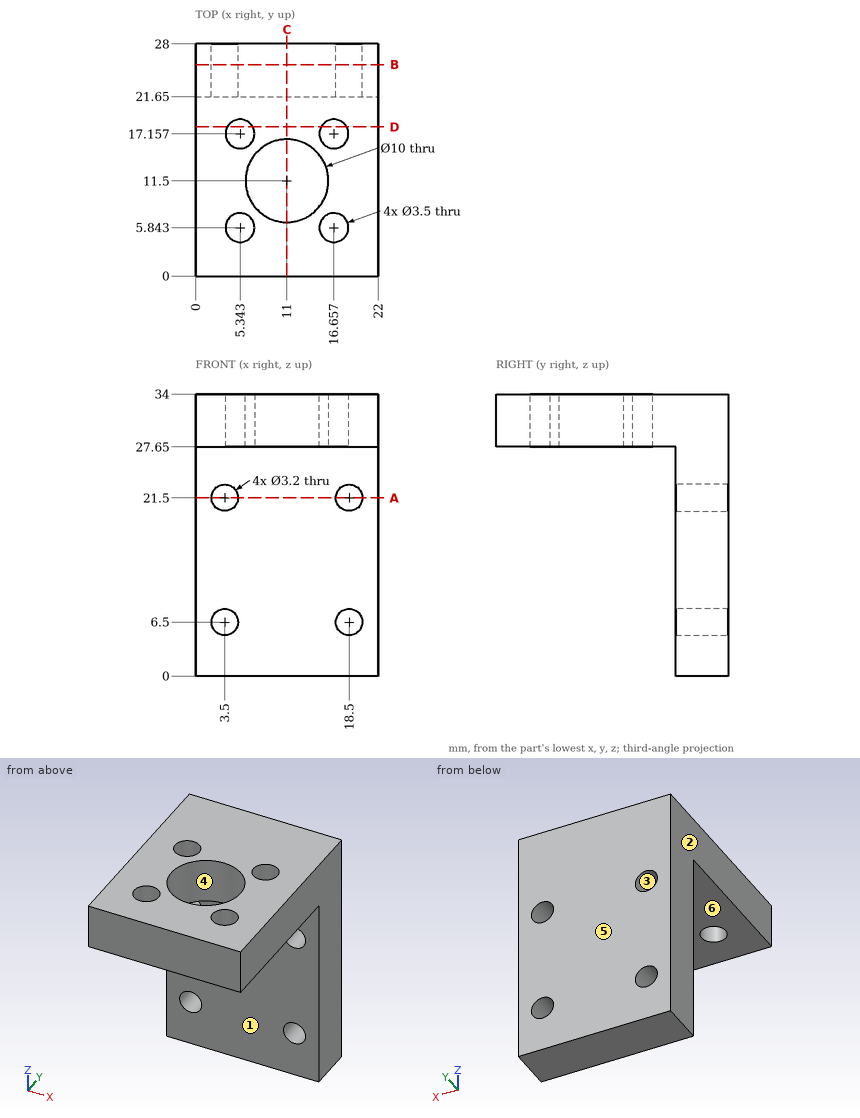
Answer from the drawing. Dimensions are ordinates in mm from the lowest x, y and z of the part. A direction names the side the tool comes from. Coordinates: 2 decimals unless noted, no trailing zeros. Loops run counter-clockwise (first coordinate to the right, second up) from the corner with the lowest first, then second, coordinate; pieces in that order, holes last. Notation, with made-up numbers: (57, 69) - (93, 69) arc R32 ccw to (93, 108) - close; hole circle Ø9 at (41.25, 15). An arc over 180 degrees is marked (long way). Use a Markdown table: item, result.
Item 1: Find section B-B, the plane y = 25.5. Determine the outline of the cut face in (x, z).
Evaluation:
| item | result |
|---|---|
| outline | (0, 0) - (22, 0) - (22, 34) - (0, 34) - close; hole circle Ø3.2 at (3.5, 6.5); hole circle Ø3.2 at (3.5, 21.5); hole circle Ø3.2 at (18.5, 6.5); hole circle Ø3.2 at (18.5, 21.5) |
Item 2: For the marked faces 5 and 6, determine the directions among +Z, -Z, +X, -X, +Y, -Y from which every point of the face is accessible in a straight line to the end or side of a thin tool.
Evaluation:
| item | result |
|---|---|
| face 5 | +Z, -Z, +X, -X, +Y |
| face 6 | -Z, +X, -X, -Y |
Item 3: Find section D-D, the plane y = 18. Determine the outline of the cut face in (x, z).
Evaluation:
| item | result |
|---|---|
| outline | (0, 27.65) - (3.81, 27.65) - (3.81, 34) - (0, 34) - close; (6.88, 27.65) - (15.12, 27.65) - (15.12, 34) - (6.88, 34) - close; (18.19, 27.65) - (22, 27.65) - (22, 34) - (18.19, 34) - close |
Item 4: Find section C-C, the plane x = 11. Determine the outline of the cut face in (y, z), and give its area (3 significant figures).
Evaluation:
| item | result |
|---|---|
| outline | (0, 27.65) - (6.5, 27.65) - (6.5, 34) - (0, 34) - close; (16.5, 27.65) - (21.65, 27.65) - (21.65, 0) - (28, 0) - (28, 34) - (16.5, 34) - close |
| area | 290 mm2 |
Item 5: Find section A-A, the plane z = 21.5. Determine the outline of the cut face in (x, y).
Evaluation:
| item | result |
|---|---|
| outline | (0, 21.65) - (1.9, 21.65) - (1.9, 28) - (0, 28) - close; (5.1, 21.65) - (16.9, 21.65) - (16.9, 28) - (5.1, 28) - close; (20.1, 21.65) - (22, 21.65) - (22, 28) - (20.1, 28) - close |
Item 6: Given pin 1 Ø5 at (x, z) = (3.5, 21.5) entering from -Y; pin 2 Ø5.5 at (x, y) = (16.66, 5.84) entering from -Z; pin 3 Ø1 at (x, y) = (8.5, 21.5) entering from -Z, each flat-ended and moving along its own axis, determine where each tip first touches the part or whether it passes through.
Evaluation:
| item | result |
|---|---|
| pin 1 | stops at y = 21.65 |
| pin 2 | stops at z = 27.65 |
| pin 3 | stops at z = 0 |
Item 7: The mould has two halves that part along X. Classify the marked faces 1, 2, 3 and 4: +X half, -X half, draft (parallel to the pull), parting line (faces both ways), or undercut.
Evaluation:
| item | result |
|---|---|
| face 1 | draft |
| face 2 | -X half |
| face 3 | undercut |
| face 4 | undercut |
Item 8: Consider probe 1 along Y at (x, z) = (5.5, 32); probe 2 along X at (y, z) = (23.5, 6.5); probe 3 along Y at (x, z) = (5.25, 18.5). Determine where each line is inside the solid, lowest interval first. Write a range as from..to.
Evaluation:
| item | result |
|---|---|
| probe 1 | y = 0..4.1, 7.59..15.41, 18.9..28 |
| probe 2 | x = 0..1.9, 5.1..16.9, 20.1..22 |
| probe 3 | y = 21.65..28 |
